from build123d import *

# Parameters (mm, degrees)
SM_BASE_FLANGE_1_DEPTH = 270
SKETCH_2_R             = 2
CUT_EXTRUDE_1_DEPTH    = 137
SKETCH_3_R             = 2
CUT_EXTRUDE_2_DEPTH    = 10


# Sheet-metal steps are written as plain solids
with BuildPart() as part:
    # Sketch 1 → Базовая кромка1 (new body)
    with BuildSketch(Plane(origin=(0, 0, 0), x_dir=(1, 0, 0), z_dir=(0, 1, 0))):
        with BuildLine():
            Line((-3.932431311, 56.4), (42.156298852, 56.4))
            ThreePointArc((42.156298852, 56.4), (42.998202403, 56.232534972), (43.71193377, 55.755634919))
            Line((43.71193377, 55.755634919), (75.834350896, 23.633217793))
            ThreePointArc((75.834350896, 23.633217793), (76.311250949, 22.919486426), (76.478715977, 22.077582874))
            Line((76.478715977, 22.077582874), (76.478715977, -22.077582874))
            ThreePointArc((76.478715977, -22.077582874), (76.311250949, -22.919486426), (75.834350896, -23.633217793))
            Line((75.834350896, -23.633217793), (43.51193377, -55.955634919))
            ThreePointArc((43.51193377, -55.955634919), (42.798202403, -56.432534972), (41.956298852, -56.6))
            Line((41.956298852, -56.6), (-4.132431311, -56.6))
            Line((-4.132431311, -56.6), (-4.132431311, -55.6))
            Line((-4.132431311, -55.6), (41.956298852, -55.6))
            ThreePointArc((41.956298852, -55.6), (42.41551897, -55.508655439), (42.804826989, -55.248528137))
            Line((42.804826989, -55.248528137), (75.127244115, -22.926111012))
            ThreePointArc((75.127244115, -22.926111012), (75.387371416, -22.536802993), (75.478715977, -22.077582874))
            Line((75.478715977, -22.077582874), (75.478715977, 22.077582874))
            ThreePointArc((75.478715977, 22.077582874), (75.387371416, 22.536802993), (75.127244115, 22.926111012))
            Line((75.127244115, 22.926111012), (43.004826989, 55.048528137))
            ThreePointArc((43.004826989, 55.048528137), (42.61551897, 55.308655439), (42.156298852, 55.4))
            Line((42.156298852, 55.4), (-3.932431311, 55.4))
            Line((-3.932431311, 55.4), (-3.932431311, 56.4))
        make_face()
    extrude(amount=SM_BASE_FLANGE_1_DEPTH)

    # Эскиз2 → Вырез-Вытянуть1 (cut)
    with BuildSketch(Plane(origin=(0, 0, -56.4), x_dir=(-1, 0, 0), z_dir=(0, 0, -1))):
        with Locations((-19.11193377, 5)):
            Circle(SKETCH_2_R)
    extrude(amount=-CUT_EXTRUDE_1_DEPTH, mode=Mode.SUBTRACT)

    # Эскиз3 → Вырез-Вытянуть2 (cut)
    with BuildSketch(Plane(origin=(76.478715977, 0, 0), x_dir=(0, 0, -1), z_dir=(1, 0, 0))):
        with Locations((0, 5)):
            Circle(SKETCH_3_R)
    extrude(amount=-CUT_EXTRUDE_2_DEPTH, mode=Mode.SUBTRACT)


solid = part.part
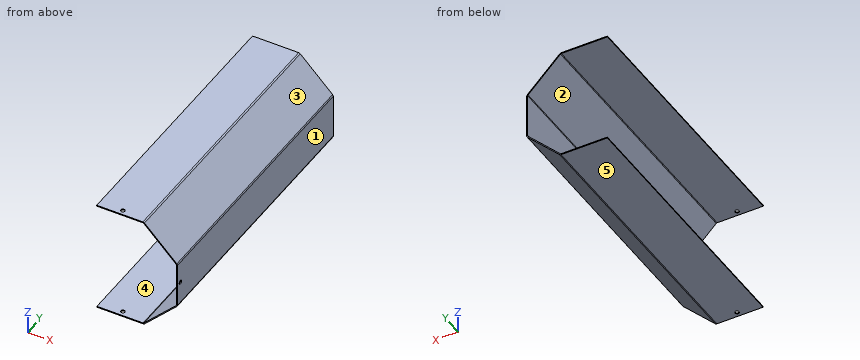
The listing builds one solid part. Answer for the finished solid, in the listing's coordinates (mm). Face numbers are marked on the shaded views. A direction names the side the tool comes from. Give positions to 0.01 mm unless a question says otherwise; leave off trailing zeros. Write each loop counter-clockwise with the first axis right and the second up, starting at its lowest first coordinate (ties: lowest second). Pieces come first, ordered by that corner, then holes. Notation, with made-up numbers: (18, 44.25) -> (77, 44.25) arc R26 cw to (77, 63.25) -> close; hole circle Ø4 at (29, -25.5). An arc over 180 degrees is marked (long way). One line per question, with ' | ' between items. Start each with the question number.
1. Section C-C (z = 6.5) is taken. Determine the outline of the cut face in (x, y).
2. Given pin 1 Ø2.5 at (y, z) = (5, 0) entering from +X; pin 2 Ø8 at (y, z) = (171.5, 34) entering from +X; pin 3 Ø3 at (y, z) = (172, -19.5) entering from -X; pin 4 Ø2 at (y, z) = (53, -44.5) entering from -X, each flat-ended and moving along its own axis, determine where each tip first touches the part or whether it passes through.
3. For the marked faces 4 and 5, determine the directions among +Z, -Z, +X, -X, +Y, -Y from which every point of the face is accessible in a straight line to the end or side of a thin tool.
4. Find the intervals of material crossed by probe 1 along Y at (x, z) = (75.9, 0); probe 2 along Z at (x, y) = (2, 232); probe 3 along X at (y, z) = (211, -4), in increasing order.
5. Section B-B (y = 218) is taken. Determine the outline of the cut face in (x, z), plus the area to 3 significant figures.
6. Section D-D (z = 34) is taken. Determine the outline of the cut face in (x, y).
7. Section A-A (x = 57) is taken. Determine the outline of the cut face in (y, z).
8. For a pull along Z with two mould halves and no side action, classify the marked faces 1, 2 and 3 as pulls with the +Z half, pulls with the -Z half, needs draft (parallel to the pull), parting line crosses it, or undercut.
Response values:
1) outline: (75.48, 0) -> (76.48, 0) -> (76.48, 270) -> (75.48, 270) -> close
2) pin 1: through | pin 2: x = 69.47 | pin 3: x = 75.48 | pin 4: x = 52.55
3) face 4: -X, +Y, -Y | face 5: -Z, +X, -X, +Y, -Y
4) probe 1: 0 to 3, 7 to 270 | probe 2: -56.4 to -55.4, 55.6 to 56.6 | probe 3: 75.48 to 76.48
5) outline: (-4.13, 55.6) -> (41.96, 55.6) arc R1.2 cw to (42.8, 55.25) -> (75.13, 22.93) arc R1.2 cw to (75.48, 22.08) -> (75.48, -22.08) arc R1.2 cw to (75.13, -22.93) -> (43, -55.05) arc R1.2 cw to (42.16, -55.4) -> (-3.93, -55.4) -> (-3.93, -56.4) -> (42.16, -56.4) arc R2.2 ccw to (43.71, -55.76) -> (75.83, -23.63) arc R2.2 ccw to (76.48, -22.08) -> (76.48, 22.08) arc R2.2 ccw to (75.83, 23.63) -> (43.51, 55.96) arc R2.2 ccw to (41.96, 56.6) -> (-4.13, 56.6) -> close | area: 233 mm2
6) outline: (64.05, 0) -> (65.47, 0) -> (65.47, 270) -> (64.05, 270) -> close
7) outline: (0, -42.47) -> (270, -42.47) -> (270, -41.05) -> (0, -41.05) -> close; (0, 41.05) -> (270, 41.05) -> (270, 42.47) -> (0, 42.47) -> close
8) face 1: needs draft | face 2: undercut | face 3: pulls with the +Z half
